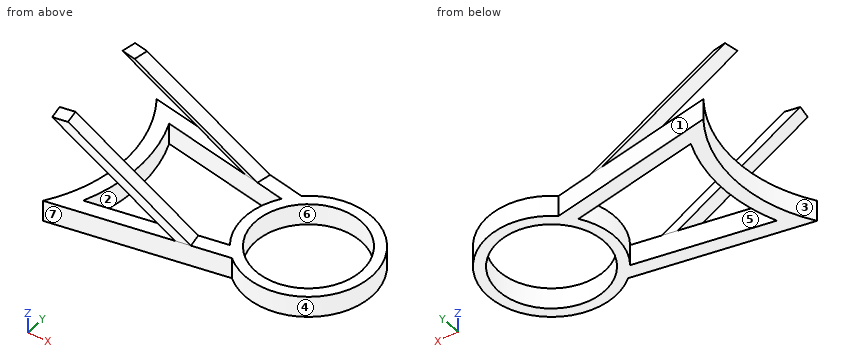
```python
from build123d import *

# Parameters (mm, degrees)
SKETCH2_R      = 375
EXTRUDE1_DEPTH = 150
EXTRUDE2_DEPTH = 1000


with BuildPart() as part:
    # Sketch2 → Extrude1 (new body)
    with BuildSketch(Plane.XY.offset(10859.457415778)):
        with BuildLine():
            Line((4595.965460825, 3982.309677998), (3420.142893862, 4198.672715486))
            ThreePointArc((3420.142893862, 4198.672715486), (3589.772208911, 3641.46133228), (3420.142893862, 3084.249949073))
            Line((3420.142893862, 3084.249949073), (4595.965460825, 3300.612986561))
            ThreePointArc((4595.965460825, 3300.612986561), (5339.772208911, 3641.46133228), (4595.965460825, 3982.309677998))
        make_face()
        with Locations((4889.772208911, 3641.46133228)):
            Circle(SKETCH2_R, mode=Mode.SUBTRACT)
        with BuildLine():
            Line((4517.981926059, 3894.980533873), (3605.871957835, 4062.817832453))
            ThreePointArc((3605.871957835, 4062.817832453), (3689.772208911, 3641.46133228), (3605.871957835, 3220.104832106))
            Line((3605.871957835, 3220.104832106), (4517.981926059, 3387.942130686))
            ThreePointArc((4517.981926059, 3387.942130686), (4439.772208911, 3641.46133228), (4517.981926059, 3894.980533873))
        make_face(mode=Mode.SUBTRACT)
    extrude(amount=EXTRUDE1_DEPTH)

    # Sketch3 → Extrude2 (add, along a direction that is not the sketch's normal)
    with BuildSketch(Plane.XY.offset(11009.457415778)):
        Polygon((4340.484797421, 4029.320658997), (4242.135965642, 4047.417821421), (4224.038803218, 3949.068989643), (4322.387634996, 3930.971827218), align=None)
        Polygon((4322.387634996, 3351.950837341), (4224.038803218, 3333.853674916), (4242.135965642, 3235.504843138), (4340.484797421, 3253.602005562), align=None)
    extrude(amount=EXTRUDE2_DEPTH, dir=(-0.866025404, 0, 0.5))


solid = part.part
```
Geometry: final body of the model. Coordinates: model frame, mm. Face numbers are marked on the shaded views. A direction names the side the tool comes from. Coordinates: 2 decimals unless noted, no trailing zeros. Order: outer loops, then holes, each group sorted by start corner. A loop starts at its lowest first (then second) coordinate and runs counter-clockwise, first axis right, second up. Notation, with made-up numbers: (-0.5, 24) -> (53.5, 24) arc R10 ccw to (53.5, 41) -> close; hole circle Ø3 at (-33.75, -11). An arc over 180 degrees is marked (long way). Use CSV: the item, a comma, the result in double quotes.
1) Section A-A on y = 3736. Output: boundary loops of the cut face in (x, z).
Findings:
outline,"(3585.29, 10859.46) -> (3685.7, 10859.46) -> (3685.7, 11009.46) -> (3585.29, 11009.46) -> close; (4449.81, 10859.46) -> (4526.88, 10859.46) -> (4526.88, 11009.46) -> (4449.81, 11009.46) -> close; (5252.66, 10859.46) -> (5329.73, 10859.46) -> (5329.73, 11009.46) -> (5252.66, 11009.46) -> close"
2) Access query for the marked faces 5, 6 and 7. Directions: +Z, -Z, +X, -X, +Y, -Y. A direction counts if a zero-diameter tool reaches every point of the face in a straight line with its end or side. Return the directions, or none.
Findings:
face 5,"-Z"
face 6,"+Z, -Z"
face 7,"+Z, -Z, -Y"
3) Section D-D on x = 5085. Output: boundary loops of the cut face in (y, z).
Findings:
outline,"(3236.02, 10859.46) -> (3321.29, 10859.46) -> (3321.29, 11009.46) -> (3236.02, 11009.46) -> close; (3961.63, 10859.46) -> (4046.91, 10859.46) -> (4046.91, 11009.46) -> (3961.63, 11009.46) -> close"
4) Section C-C on x = 3795. Output: boundary loops of the cut face in (y, z), then the cut area to 3 significant figures.
Findings:
outline,"(3153.23, 10859.46) -> (3254.91, 10859.46) -> (3254.91, 11009.46) -> (3153.23, 11009.46) -> close; (3235.5, 11267.61) -> (3333.85, 11257.16) -> (3351.95, 11313.94) -> (3253.6, 11324.39) -> close; (3930.97, 11313.94) -> (3949.07, 11257.16) -> (4047.42, 11267.61) -> (4029.32, 11324.39) -> close; (4028.02, 10859.46) -> (4129.7, 10859.46) -> (4129.7, 11009.46) -> (4028.02, 11009.46) -> close"
area,"42,100 mm^2"
5) Section B-B on z = 11319.5. Output: boundary loops of the cut face in (x, y), then the cut area to 3 significant figures.
Findings:
outline,"(3687.03, 3333.85) -> (3705.13, 3235.5) -> (3803.48, 3253.6) -> (3785.38, 3351.95) -> close; (3687.03, 3949.07) -> (3785.38, 3930.97) -> (3803.48, 4029.32) -> (3705.13, 4047.42) -> close"
area,"20,000 mm^2"
6) Line query: line 1 (Z direction, x = 3671.5, y = 3649.5); line 2 (Z direction, x = 4009, y = 3990); line 3 (Y direction, x = 4096, z = 11094). Output: solid intervals per line, ascending.
Findings:
line 1,"z = 10859.46 to 11009.46"
line 2,"z = 10859.46 to 11009.46, 11137.96 to 11196.66"
line 3,"y = 3235.56 to 3337.24, 3945.68 to 4047.36"
7) Pin query (flat end, axial travel): pin 1 Ø5 at (x, z) = (4769, 10967.5) entering from +Y; pin 2 Ø1 at (x, z) = (4739.5, 10953.5) entering from -Y; pin 3 Ø8 at (x, y) = (4068, 3225) entering from +Z. Return the tip coordinate at first contact, or that it passes through.
Findings:
pin 1,"stops at y = 4075.64"
pin 2,"stops at y = 3217.12"
pin 3,"stops at z = 11009.46"
8) Mould query, pull axis Y, two halves, no side actions, for the marked faces 1, 2, 3 and 4. Classes: +Y half, -Y half, draft (parallel to the pull), parting line (faces both ways), or undercut.
Findings:
face 1,"+Y half"
face 2,"undercut"
face 3,"undercut"
face 4,"parting line"
